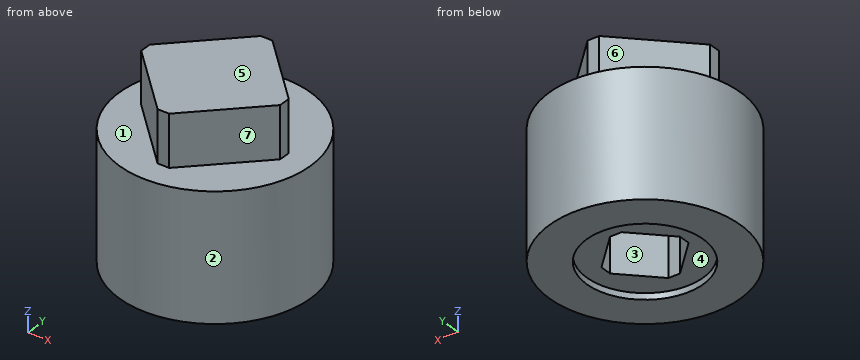
```python
from build123d import *

# Parameters (mm, degrees)
REPLACEABLE_START                           = 1
SKETCH1_R                                   = 16.7
REPLACEABLE_DRIVE_INSERT_BODY_DEPTH         = 22
COMMON_START                                = 23
COMMON_POSITIVE_DRIVE_TANG_DEPTH            = 9
VALVE_START                                 = 1
VALVE_STEM_SOCKET_NOMINAL_FLATS_11_MM_DEPTH = 19.1
STEM_START                                  = 1
SKETCH4_R                                   = 10.2
STEM_CORNER_CLEARANCE_AT_ENTRY_DEPTH        = 1.1


with BuildPart() as part:
    # Sketch1 → Replaceable drive insert body (new body)
    with BuildSketch(Plane.XY.offset(REPLACEABLE_START)):
        Circle(SKETCH1_R)
    extrude(amount=REPLACEABLE_DRIVE_INSERT_BODY_DEPTH)

    # Sketch2 → Common positive drive tang (add)
    with BuildSketch(Plane.XY.offset(COMMON_START)):
        Polygon((1.02, 12.202896808), (-1.02, 12.202896808), (-12.202896808, 1.02), (-12.202896808, -1.02), (-1.02, -12.202896808), (1.02, -12.202896808), (12.202896808, -1.02), (12.202896808, 1.02), align=None)
    extrude(amount=COMMON_POSITIVE_DRIVE_TANG_DEPTH)

    # Sketch3 → Valve stem socket, nominal flats 11 mm (cut)
    with BuildSketch(Plane.XY.offset(VALVE_START)):
        Polygon((1.02, 6.899595949), (-1.02, 6.899595949), (-6.899595949, 1.02), (-6.899595949, -1.02), (-1.02, -6.899595949), (1.02, -6.899595949), (6.899595949, -1.02), (6.899595949, 1.02), align=None)
    extrude(amount=VALVE_STEM_SOCKET_NOMINAL_FLATS_11_MM_DEPTH, mode=Mode.SUBTRACT)

    # Sketch4 → Stem corner clearance at entry (cut)
    with BuildSketch(Plane.XY.offset(STEM_START)):
        Circle(SKETCH4_R)
    extrude(amount=STEM_CORNER_CLEARANCE_AT_ENTRY_DEPTH, mode=Mode.SUBTRACT)


solid = part.part
```
The listing builds one solid part. Answer for the finished solid, in the listing's coordinates (mm). Face numbers are marked on the shaded views. A direction names the side the tool comes from. Coordinates: 2 decimals unless noted, no trailing zeros. Loops run counter-clockwise (first coordinate to the right, second up) from the corner with the lowest first, then second, coordinate; pieces in that order, holes last. Notation, with made-up numbers: (30, -15.75) -> (86, -15.75) arc R24 cw to (86, 8.25) -> close; hole circle Ø2 at (86, 3). An arc over 180 degrees is marked (long way). Return JSON: item names as keys, results as strings. Group by question number.
(1) Find the intervals of material crossed by probe 1 along Y at (x, z) = (0, 1.35); probe 2 along Z at (x, y) = (13.5, 3.5); probe 3 along X at (y, z) = (0.5, 14), in increasing order. Write a range as from..to.
(2) A cutting plane is placed at A-A on z = 25.5. Write down the section's boundary in (x, y), and give its area (3 significant figures).
(3) Determine the mould class of the marked faces 1, 2 and 3 for opening direction Y: released by +Y, released by -Y, zero draft, split by the parting line, or undercut.
(4) Given pin 1 Ø0.6 at (x, z) = (0, 28) entering from -Y; pin 2 Ø0.6 at (y, z) = (-0.5, 26.5) entering from -X; pin 3 Ø11 at (x, y) = (-3.5, -1.5) entering from -Z; pin 4 Ø1.5 at (x, y) = (-13, 13) entering from +Z, each flat-ended and moving along its own axis, determine where each tip first touches the part or whether it passes through.
(5) A cutting plane is placed at D-D on z = 10.5. Write down the section's boundary in (x, y), and give its area (3 significant figures).
(6) Which of the six approach directions +Z, -Z, +X, -X, +Y, -Y give full straight-line access (tool end or side, diameter ignored) to the marked faces 4, 5, 6 and 7?
(7) A cutting plane is placed at B-B on y = 0. Write down the section's boundary in (x, z), and give its area (3 significant figures).
The answers:
{
 "1": {"probe 1": "y = -16.7..-10.2, 10.2..16.7", "probe 2": "z = 1..23", "probe 3": "x = -16.69..-6.9, 6.9..16.69"},
 "2": {"outline": "(-12.2, -1.02) -> (-1.02, -12.2) -> (1.02, -12.2) -> (12.2, -1.02) -> (12.2, 1.02) -> (1.02, 12.2) -> (-1.02, 12.2) -> (-12.2, 1.02) -> close", "area": "346 mm^2"},
 "3": {"face 1": "zero draft", "face 2": "split by the parting line", "face 3": "undercut"},
 "4": {"pin 1": "stops at y = -12.2", "pin 2": "stops at x = -12.2", "pin 3": "stops at z = 2.1", "pin 4": "passes through"},
 "5": {"outline": "circle Ø33.4 at (0, 0); hole (-6.9, -1.02) -> (-1.02, -6.9) -> (1.02, -6.9) -> (6.9, -1.02) -> (6.9, 1.02) -> (1.02, 6.9) -> (-1.02, 6.9) -> (-6.9, 1.02) -> close", "area": "755 mm^2"},
 "6": {"face 4": "-Z", "face 5": "+Z, +X, -X, +Y, -Y", "face 6": "+Z, -X, +Y", "face 7": "+Z, +X, -Y"},
 "7": {"outline": "(-16.7, 1) -> (-10.2, 1) -> (-10.2, 2.1) -> (-6.9, 2.1) -> (-6.9, 20.1) -> (6.9, 20.1) -> (6.9, 2.1) -> (10.2, 2.1) -> (10.2, 1) -> (16.7, 1) -> (16.7, 23) -> (12.2, 23) -> (12.2, 32) -> (-12.2, 32) -> (-12.2, 23) -> (-16.7, 23) -> close", "area": "684 mm^2"}
}
